Build history of the part. All positions in model axes, mm. Face numbers are marked on the shaded views. A direction names the side the tool comes from. Coordinates: 2 decimals unless noted, no trailing zeros. Loops run counter-clockwise (first coordinate to the right, second up) from the corner with the lowest first, then second, coordinate; pieces in that order, holes last. Notation, with made-up numbers: M -13,-24.75 L 32,-24.75 A25 cw 32,-8.75 Z; hole C 30,-3 d7. An arc over 180 degrees is marked long. Write each question's results on one line, items separated by ' | '. Start each with the question number.
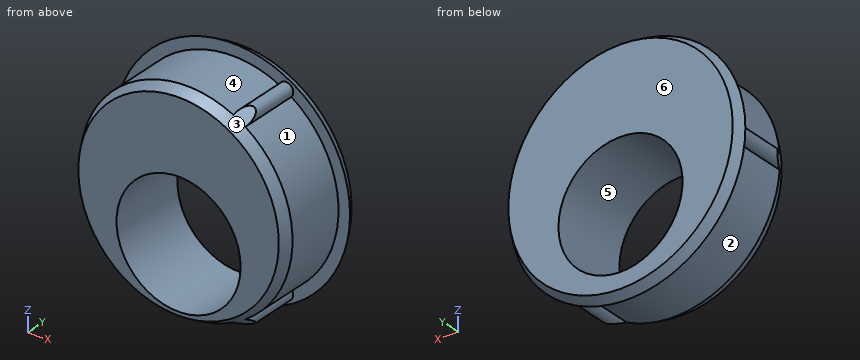
from build123d import *

# Parameters (mm, degrees)
F0_R          = 22.25
F0_R_2        = 13
F1_DEPTH      = 15
F1_DEPTH_BACK = 2
F4_R          = 1.5
F5_DEPTH      = 15


with BuildPart() as f1:
    # F0 (on Front) → F1 (new body, two sides)
    with BuildSketch(Plane.XZ) as f1_sk:
        Circle(F0_R)
        with Locations((0, -7.25)):
            Circle(F0_R_2, mode=Mode.SUBTRACT)
    extrude(amount=F1_DEPTH)
    extrude(f1_sk.sketch, amount=-F1_DEPTH_BACK)

    # F2 (on Top) → F3 (revolve)
    with BuildSketch(Plane.XY):
        Polygon((-24.6547005384, 0), (-21.5, 0), (-21.5, 2), (-23.5, 2), align=None)
    revolve(axis=Axis((0, 0, 0), (0, 1, 0)))

    # F4 (on Front) → F5 (join, through all)
    with BuildSketch(Plane.XZ):
        with Locations((-22.5, 0)):
            Circle(F4_R)
        with Locations((11.25, -19.4855715851)):
            Circle(F4_R)
        with Locations((11.25, 19.4855715851)):
            Circle(F4_R)
    extrude(amount=F5_DEPTH)

    # F6 (on Top) → F7 (revolve, cut)
    with BuildSketch(Plane.XY):
        Polygon((-24.8129580218, -15), (-21, -15), (-24.8129580218, -8.3957629791), align=None)
    revolve(axis=Axis((0, 0, 0), (0, 1, 0)), mode=Mode.SUBTRACT)


solid = f1.part
1. Band-saw the part on A-A, the plane x = 0. List the corners of the cut face in (y, z), plus the area to 3 significant figures.
2. Band-saw the part on C-C, the plane y = -4. List the corners of the cut face in (x, z).
3. Pin check, flat tips, straight feed: pin 1 (10 mm diameter, centred on y = -6.5, z = 7.5, fed in from -X); pin 2 (3 mm diameter, centred on x = -18, y = -6, fed in from -Z); pin 3 (1.5 mm diameter, centred on x = 11, y = -4.5, fed in from -Z). Stop position of each tip, or through.
4. Mould opens along Z. For the marked faces 4, 5 and 6 say: +Z half, -Z half, draft (parallel to the pull), parting line (faces both ways), or undercut.
5. Which spindle directions (+Z, -Z, +X, -X, +Y, -Y) get a long thin tool onto all of the face, cutting with end or side? Do the marked faces 1, 2 and 3. Say none if no direction does.
6. Wall check: line 1 along Z through (x, y) = (0, -5.25); line 2 along X through (y, z) = (-6, -18.5); line 3 along Z through (x, y) = (-8, -13). Give the ranges that are in metal, low to high.
7. Band-saw the part on B-B, the plane y = -11. List the corners of the cut face in (x, z), plus the area to 3 significant figures.
Checked values:
1) outline: M -15,-21 L -12.83,-22.25 L 0,-22.25 L 0,-24.65 L 2,-23.5 L 2,-20.25 L -15,-20.25 Z; M -15,5.75 L 2,5.75 L 2,23.5 L 0,24.65 L 0,22.25 L -12.83,22.25 L -15,21 Z | area: 319 mm²
2) outline: M -22.2,-1.47 A22.25 ccw 9.83,-19.96 A1.5 ccw long 12.37,-18.49 A22.25 ccw 12.37,18.49 A1.5 ccw long 9.83,19.96 A22.25 ccw -22.2,1.47 A1.5 ccw long Z; hole C 0,-7.25 d26
3) pin 1: x = -22.11 | pin 2: z = -14.93 | pin 3: z = -20.99
4) face 4: +Z half | face 5: undercut | face 6: draft
5) face 1: +X, -Y | face 2: -Z, -Y | face 3: -Y
6) line 1: -22.25 to -20.25, 5.75 to 22.25 | line 2: -12.36 to -6.51, 6.51 to 12.38 | line 3: -20.66 to -17.5, 3 to 20.66
7) outline: M -23.27,-1.28 A1.5 ccw -22.2,-1.47 A22.25 ccw 9.83,-19.96 A1.5 ccw 10.52,-20.8 A23.31 ccw 12.75,-19.51 A1.5 ccw 12.37,-18.49 A22.25 ccw 12.37,18.49 A1.5 ccw 12.75,19.51 A23.31 ccw 10.52,20.8 A1.5 ccw 9.83,19.96 A22.25 ccw -22.2,1.47 A1.5 ccw -23.27,1.28 A23.31 ccw Z; hole C 0,-7.25 d26 | area: 1,030 mm²
